Read the model definition and answer for the solid it produces. Units are mm, in the model's axes. Face numbers are marked on the shaded views. A direction names the side the tool comes from. Give positions to 0.01 mm unless a question says otherwise; leave off trailing zeros. Write each loop counter-clockwise with the first axis right and the second up, starting at its lowest first coordinate (ties: lowest second). Pieces come first, ordered by that corner, then holes. Notation, with made-up numbers: (71, 70) - (80, 70) arc R24 ccw to (80, 107) - close; hole circle Ø10 at (17, 2). An arc over 180 degrees is marked (long way). Use CSV: the item, a comma, the result in double quotes. Start each with the question number.
from build123d import *

# Parameters (mm, degrees)
SKETCH004_W     = 27
SKETCH004_H     = 27.3
PAD005_DEPTH    = 1
POCKET003_DEPTH = 1.001
SKETCH005_W     = 27
SKETCH005_H     = 19
PAD001_DEPTH    = 1.6
SKETCH006_R     = 0.9
PAD006_DEPTH    = 0.5


with BuildPart() as part:
    # Sketch004 → Pad005 (new body)
    with BuildSketch(Plane.XY):
        with Locations((13.5, 13.65)):
            Rectangle(SKETCH004_W, SKETCH004_H)
    extrude(amount=PAD005_DEPTH)

    # Sketch001 → Pocket003 (cut, through all)
    with BuildSketch(Plane.XY.offset(1)):
        with BuildLine():
            ThreePointArc((1.75, 26.3), (0.625, 25.175), (1.75, 24.05))
            Line((1.75, 24.05), (3, 24.05))
            ThreePointArc((3, 24.05), (4.125, 25.175), (3, 26.3))
            Line((1.75, 26.3), (3, 26.3))
        make_face()
        with BuildLine():
            ThreePointArc((24, 26.3), (22.875, 25.175), (24, 24.05))
            Line((24, 24.05), (25.25, 24.05))
            ThreePointArc((25.25, 24.05), (26.375, 25.175), (25.25, 26.3))
            Line((24, 26.3), (25.25, 26.3))
        make_face()
        with BuildLine():
            ThreePointArc((1.75, 3.25), (0.625, 2.125), (1.75, 1))
            Line((1.75, 1), (3, 1))
            ThreePointArc((3, 1), (4.125, 2.125), (3, 3.25))
            Line((1.75, 3.25), (3, 3.25))
        make_face()
        with BuildLine():
            ThreePointArc((24, 3.25), (22.875, 2.125), (24, 1))
            Line((24, 1), (25.25, 1))
            ThreePointArc((25.25, 1), (26.375, 2.125), (25.25, 3.25))
            Line((24, 3.25), (25.25, 3.25))
        make_face()
    extrude(amount=-POCKET003_DEPTH, mode=Mode.SUBTRACT)

    # Sketch005 → Pad001 (new body)
    with BuildSketch(Plane.XY.offset(1)):
        with Locations((13.5, 13.6)):
            Rectangle(SKETCH005_W, SKETCH005_H)
    extrude(amount=PAD001_DEPTH)

    # Sketch006 → Pad006 (new body)
    with BuildSketch(Plane.XY.offset(1)):
        with Locations((9.5, 25.55)):
            Circle(SKETCH006_R)
        with Locations((11.95, 25.55)):
            Circle(SKETCH006_R)
        with Locations((14.4, 25.55)):
            Circle(SKETCH006_R)
        with Locations((16.85, 25.55)):
            Circle(SKETCH006_R)
    extrude(amount=PAD006_DEPTH)


solid = part.part
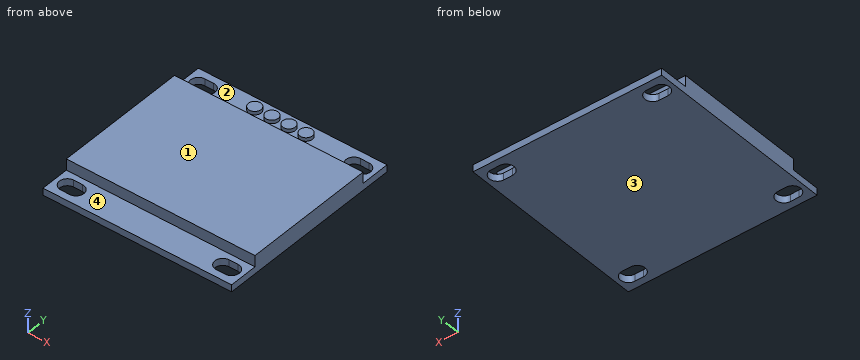
(1) Given P1, Ø1.3, axis at x = 9, z = 1.5, coming from the -Y side; P2, Ø1.4, axis at x = 12, y = 25.5, coming from the +Z side; P3, Ø1.2, axis at x = 7.5, y = 1.5, coming from the +Z side, each flat-ended and moving along its own axis, determine where each tip first touches the part or whether it passes through.
(2) Consider probe 1 along Y at (x, z) = (3, 0.7); probe 2 along Y at (x, z) = (19.5, 1.2); probe 3 along Z at (x, y) = (20.25, 26.25). Determine where each line is inside the solid, lowest interval first.
(3) For a pull along Y with two mould halves and no side action, classify the marked faces 1 and 2 as pulls with the +Y half, pulls with the -Y half, needs draft (parallel to the pull), parting line crosses it, or undercut.
(4) The part is cut by section A-A on z = 0.6. Write down the section's boundary in (x, y) (3 decimals).
(5) The part is cut by section D-D on x = 16.5. Write down the section's boundary in (y, z).
(6) Which of the six approach directions +Z, -Z, +X, -X, +Y, -Y give full straight-line access (tool end or side, diameter ignored) to the marked faces 3 and 4?
(7) The part is cut by section C-C on z = 2.2. Write down the section's boundary in (x, y), plus the area to 3 significant figures.
(8) The part is cut by section B-B on x = 9.5. Write down the section's boundary in (y, z), plus the area to 3 significant figures.
Reported:
1,P1,"y = 0"
1,P2,"z = 1.5"
1,P3,"z = 1"
2,probe 1,"0 to 1, 3.25 to 24.05, 26.3 to 27.3"
2,probe 2,"4.1 to 23.1"
2,probe 3,"0 to 1"
3,face 1,"needs draft"
3,face 2,"undercut"
4,outline,"(0, 0) - (27, 0) - (27, 27.3) - (0, 27.3) - close; hole (1.75, 1) - (3, 1) arc R1.125 ccw to (3, 3.25) - (1.75, 3.25) arc R1.125 ccw to start; hole (1.75, 24.05) - (3, 24.05) arc R1.125 ccw to (3, 26.3) - (1.75, 26.3) arc R1.125 ccw to start; hole (24, 1) - (25.25, 1) arc R1.125 ccw to (25.25, 3.25) - (24, 3.25) arc R1.125 ccw to start; hole (24, 24.05) - (25.25, 24.05) arc R1.125 ccw to (25.25, 26.3) - (24, 26.3) arc R1.125 ccw to start"
5,outline,"(0, 0) - (27.3, 0) - (27.3, 1) - (26.38, 1) - (26.38, 1.5) - (24.72, 1.5) - (24.72, 1) - (23.1, 1) - (23.1, 2.6) - (4.1, 2.6) - (4.1, 1) - (0, 1) - close"
6,face 3,"-Z, +X, -X, +Y, -Y"
6,face 4,"+Z, +X, -X, -Y"
7,outline,"(0, 4.1) - (27, 4.1) - (27, 23.1) - (0, 23.1) - close"
7,area,"513 mm²"
8,outline,"(0, 0) - (27.3, 0) - (27.3, 1) - (26.45, 1) - (26.45, 1.5) - (24.65, 1.5) - (24.65, 1) - (23.1, 1) - (23.1, 2.6) - (4.1, 2.6) - (4.1, 1) - (0, 1) - close"
8,area,"58.6 mm²"
